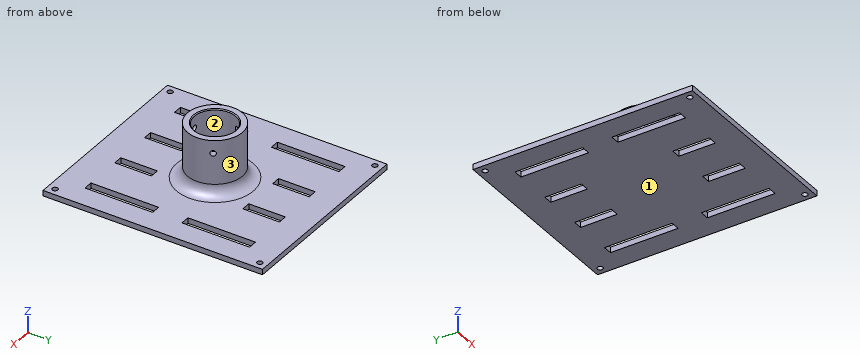
Autodesk Fusion 360 part; units mm, degrees
sketch "Sketch1" plane through (0, 0, 0) normal (0, 0, 1) x (1, 0, 0)
  line L0 (-52.2, -60) -> (52.2, -60)
  line L1 (52.2, -60) -> (52.2, 60)
  line L2 (52.2, 60) -> (-52.2, 60)
  line L3 (-52.2, 60) -> (-52.2, -60)
  dimension "d1" = 104.4
  dimension "d2" = 120
  dimension "d3" = 60
  dimension "d4" = 52.2
extrude "Extrude1" add sketch "Sketch1" along normal blind 3
sketch "Sketch2" plane through (0, 0, 3) normal (0, 0, 1) x (-1, 0, 0)
  line L0 (52.2, -60) -> (52.2, 60)
  line L1 (52.2, 60) -> (-52.2, 60)
  line L2 (-52.2, 60) -> (-52.2, -60)
  line L3 (-52.2, -60) -> (52.2, -60)
  circle A0 centre (-48.2, -56) radius 1.5
  circle A1 centre (48.2, -56) radius 1.5
  circle A2 centre (48.2, 56) radius 1.5
  circle A3 centre (-48.2, 56) radius 1.5
  dimension "d7" = 3
  dimension "d8" = 3
  dimension "d9" = 3
  dimension "d10" = 3
  dimension "d11" = 4
  dimension "d12" = 4
  dimension "d13" = 4
  dimension "d14" = 4
  dimension "d15" = 4
  dimension "d16" = 4
  dimension "d17" = 4
  dimension "d18" = 4
hole "Hole1" at (-48.2, 56, 3) at (48.2, 56, 3) at (48.2, -56, 3) at (-48.2, -56, 3) direction (0, 0, -1) diameter 3 depth 3 tip angle 118
sketch "Sketch4" plane through (0, 0, 3) normal (0, 0, 1) x (-1, 0, 0)
  circle A0 centre (-48.2, 56) radius 1.5
  circle A1 centre (48.2, -56) radius 1.5
  circle A2 centre (-48.2, -56) radius 1.5
  circle A3 centre (48.2, 56) radius 1.5
  line L0 (52.2, -60) -> (52.2, 60)
  line L1 (52.2, 60) -> (-52.2, 60)
  line L2 (-52.2, 60) -> (-52.2, -60)
  line L3 (-52.2, -60) -> (52.2, -60)
  line L4 (40, -45) -> (35, -45)
  line L5 (35, -45) -> (35, 45)
  line L6 (35, 45) -> (40, 45)
  line L7 (40, 45) -> (40, -45)
  line L8 (10, -45) -> (10, 45)
  line L9 (10, 45) -> (15, 45)
  line L10 (15, 45) -> (15, -45)
  line L11 (15, -45) -> (10, -45)
  line L12 (-15, -45) -> (-15, 45)
  line L13 (-15, 45) -> (-10, 45)
  line L14 (-10, 45) -> (-10, -45)
  line L15 (-10, -45) -> (-15, -45)
  line L16 (-40, -45) -> (-40, 45)
  line L17 (-40, 45) -> (-35, 45)
  line L18 (-35, 45) -> (-35, -45)
  line L19 (-35, -45) -> (-40, -45)
  dimension "d39" = -75
  dimension "d40" = 0
  dimension "d41" = 5
  dimension "d42" = 90
  dimension "d43" = 40
  dimension "d44" = 45
extrude "Extrude2" cut sketch "Sketch4" against normal blind 3 contours L4 L5 L6 L7 | L8 L9 L10 L11 | L12 L13 L14 L15 | L16 L17 L18 L19
sketch "Sketch6" plane through (0, 0, 3) normal (0, 0, 1) x (-1, 0, 0)
  line L0 (10, 45) -> (15, 45)
  line L1 (15, 45) -> (15, -45)
  line L2 (15, -45) -> (10, -45)
  line L3 (10, -45) -> (10, 45)
  line L4 (-15, 45) -> (-10, 45)
  line L5 (-10, 45) -> (-10, -45)
  line L6 (-10, -45) -> (-15, -45)
  line L7 (-15, -45) -> (-15, 45)
  line L8 (35, -45) -> (35, 45)
  line L9 (35, 45) -> (40, 45)
  line L10 (40, 45) -> (40, -45)
  line L11 (40, -45) -> (35, -45)
  line L12 (-40, 45) -> (-35, 45)
  line L13 (-35, 45) -> (-35, -45)
  line L14 (-35, -45) -> (-40, -45)
  line L15 (-40, -45) -> (-40, 45)
  circle A0 centre (-48.2, 56) radius 1.5
  circle A1 centre (48.2, -56) radius 1.5
  circle A2 centre (-48.2, -56) radius 1.5
  circle A3 centre (48.2, 56) radius 1.5
  line L16 (52.2, -60) -> (52.2, 60)
  line L17 (52.2, 60) -> (-52.2, 60)
  line L18 (-52.2, 60) -> (-52.2, -60)
  line L19 (-52.2, -60) -> (52.2, -60)
  line L20 (-15, 25) -> (15, 25)
  line L21 (15, 25) -> (15, -25)
  line L22 (15, -25) -> (-15, -25)
  line L23 (-15, -25) -> (-15, 25)
  line L24 (-15, 25) -> (15, -25) construction
  line L25 (15, 25) -> (-15, -25) construction
  line L26 (40, -8) -> (35, -8)
  line L27 (35, -8) -> (35, 8)
  line L28 (35, 8) -> (40, 8)
  line L29 (40, 8) -> (40, -8)
  line L30 (-35, -8) -> (-40, -8)
  line L31 (-40, -8) -> (-40, 8)
  line L32 (-40, 8) -> (-35, 8)
  line L33 (-35, 8) -> (-35, -8)
  dimension "d49" = 50
  dimension "d56" = 8
  dimension "d57" = 16
  dimension "d58" = 8
  dimension "d59" = 16
extrude "Extrude3" add sketch "Sketch6" against normal blind 3 contours L1 L3 L20 L21 L22 | L5 L7 L20 L22 L23 | L8 L10 L26 L27 L28 L29 | L13 L15 L30 L31 L32 L33
sketch "Sketch5" plane through (0, 0, 3) normal (0, 0, 1) x (-1, 0, 0)
  line L0 (10, 45) -> (15, 45)
  line L1 (15, 45) -> (15, 25)
  line L2 (15, -45) -> (10, -45)
  line L3 (10, 25) -> (10, 45)
  line L4 (-15, 45) -> (-10, 45)
  line L5 (-10, -25) -> (-10, -45)
  line L6 (-10, -45) -> (-15, -45)
  line L7 (-15, -45) -> (-15, -25)
  line L8 (35, 8) -> (35, 45)
  line L9 (35, 45) -> (40, 45)
  line L10 (40, 45) -> (40, 8)
  line L11 (40, -45) -> (35, -45)
  line L12 (-40, 45) -> (-35, 45)
  line L13 (-35, 45) -> (-35, 8)
  line L14 (-35, -45) -> (-40, -45)
  line L15 (-40, 8) -> (-40, 45)
  circle A0 centre (-48.2, 56) radius 1.5
  circle A1 centre (48.2, -56) radius 1.5
  circle A2 centre (-48.2, -56) radius 1.5
  circle A3 centre (48.2, 56) radius 1.5
  line L16 (52.2, -60) -> (52.2, 60)
  line L17 (52.2, 60) -> (-52.2, 60)
  line L18 (-52.2, 60) -> (-52.2, -60)
  line L19 (-52.2, -60) -> (52.2, -60)
  circle A4 centre (0, 0) radius 11.25
  circle A5 centre (0, 0) radius 15
  line L20 (15, 25) -> (10, 25)
  line L21 (-15, -25) -> (-10, -25)
  line L22 (10, -25) -> (15, -25)
  line L23 (15, -25) -> (15, -45)
  line L24 (10, -45) -> (10, -25)
  line L25 (-10, 25) -> (-15, 25)
  line L26 (-15, 25) -> (-15, 45)
  line L27 (-10, 45) -> (-10, 25)
  line L28 (-35, 8) -> (-40, 8)
  line L29 (40, 8) -> (35, 8)
  line L30 (35, -8) -> (40, -8)
  line L31 (40, -8) -> (40, -45)
  line L32 (35, -45) -> (35, -8)
  line L33 (-40, -8) -> (-35, -8)
  line L34 (-35, -8) -> (-35, -45)
  line L35 (-40, -45) -> (-40, -8)
  dimension "d47" = 22.5
  dimension "d48" = 30
extrude "Extrude4" add sketch "Sketch5" along normal blind 30 contours A5
fillet "Fillet1" radius 6 1 edges at (13.9849, -5.4242, 3)
chamfer "Chamfer1" distance 0.5 angle 45 1 edges at (10.4887, -4.0682, 33)
sketch "Sketch7" plane through (0, 0, 0) normal (0, 1, 0) x (1, 0, 0)
  circle A0 centre (-0.0436, -26) radius 1.5
  dimension "d61" = 26
  dimension "d62" = 3
hole "Hole3" at (-0.0436, 0, 26) direction (0, -1, 0) diameter 3 depth 17 tip angle 118
thread "Thread1"
pattern_circular "C-Pattern1" count 3 over 360 about axis through (0, 0, 1.75) along (0, 0, 1) of "Hole3"
Verification items for the finished model (mm, model axes). Face numbers are marked on the shaded views. Give positions to 0.01 mm unless a question says otherwise; leave off trailing zeros. Loops run counter-clockwise (first coordinate to the right, second up) from the corner with the lowest first, then second, coordinate; pieces in that order, holes last.
1) Draft check along Y on the marked faces 1, 2 and 3. Enter one of: pulls with the +Y half, pulls with the -Y half, needs draft (parallel to the pull), parting line crosses it, or undercut.
2) Depth check by flat-ended pin: pin 1 Ø3.5 at (x, z) = (-0.04, 26) entering from -Y; pin 2 Ø10 at (x, z) = (11, 26) entering from -Y; pin 3 Ø5 at (x, z) = (5, 20.5) entering from +Y. Enter the tip coordinate at first touch or a pass-through.
3) Sectioned sample at A-A, the plane y = 56. Enter the section's corners in (x, z).
4) Sectioned sample at D-D, the plane z = 12. Enter the section's corners in (x, y).
5) Sectioned sample at C-C, the plane y = 31. Enter the section's corners in (x, z).
6) Thickness scan on line 1 along X through (y, z) = (56, 1); line 2 along Y through (x, z) = (48.2, 0.7); line 3 along Y through (x, z) = (0, 23). Record the ranges inside material, lowest first.
7) Sectioned sample at B-B, the plane x = 48.2. Enter the section's corners in (y, z).
Answers:
1. face 1: needs draft
1. face 2: undercut
1. face 3: parting line crosses it
2. pin 1: stops at y = -15
2. pin 2: stops at y = -13.75
2. pin 3: stops at y = 14.79
3. outline: (-52.2, 0) - (-49.7, 0) - (-49.7, 3) - (-52.2, 3) - close; (-46.7, 0) - (46.7, 0) - (46.7, 3) - (-46.7, 3) - close; (49.7, 0) - (52.2, 0) - (52.2, 3) - (49.7, 3) - close
4. outline: circle Ø30 at (0, 0); hole circle Ø22.5 at (0, 0)
5. outline: (-52.2, 0) - (-40, 0) - (-40, 3) - (-52.2, 3) - close; (-35, 0) - (-15, 0) - (-15, 3) - (-35, 3) - close; (-10, 0) - (10, 0) - (10, 3) - (-10, 3) - close; (15, 0) - (35, 0) - (35, 3) - (15, 3) - close; (40, 0) - (52.2, 0) - (52.2, 3) - (40, 3) - close
6. line 1: x = -52.2 to -49.7, -46.7 to 46.7, 49.7 to 52.2
6. line 2: y = -60 to -57.5, -54.5 to 54.5, 57.5 to 60
6. line 3: y = -15 to -11.25, 11.25 to 15
7. outline: (-60, 0) - (-57.5, 0) - (-57.5, 3) - (-60, 3) - close; (-54.5, 0) - (54.5, 0) - (54.5, 3) - (-54.5, 3) - close; (57.5, 0) - (60, 0) - (60, 3) - (57.5, 3) - close
